Input: dimensioned drawing with shaded views. Units: mm. Origin: part minimum x, y, z. A direction names the side the tool comes from. Round coordinates to 2 decimals unless told otherwise and drop trailing zeros. Loops run counter-clockwise (first coordinate to the right, second up) from the corner with the lowest first, then second, coordinate; pieces in that order, holes last. Notation, with made-up numbers: (71.25, -3.75) - (115.25, -3.75) arc R16 cw to (115.25, 4.25) - close; hole circle Ø4 at (2, 44). An arc over 180 degrees is marked (long way). One line per question, with ' | ' between items.
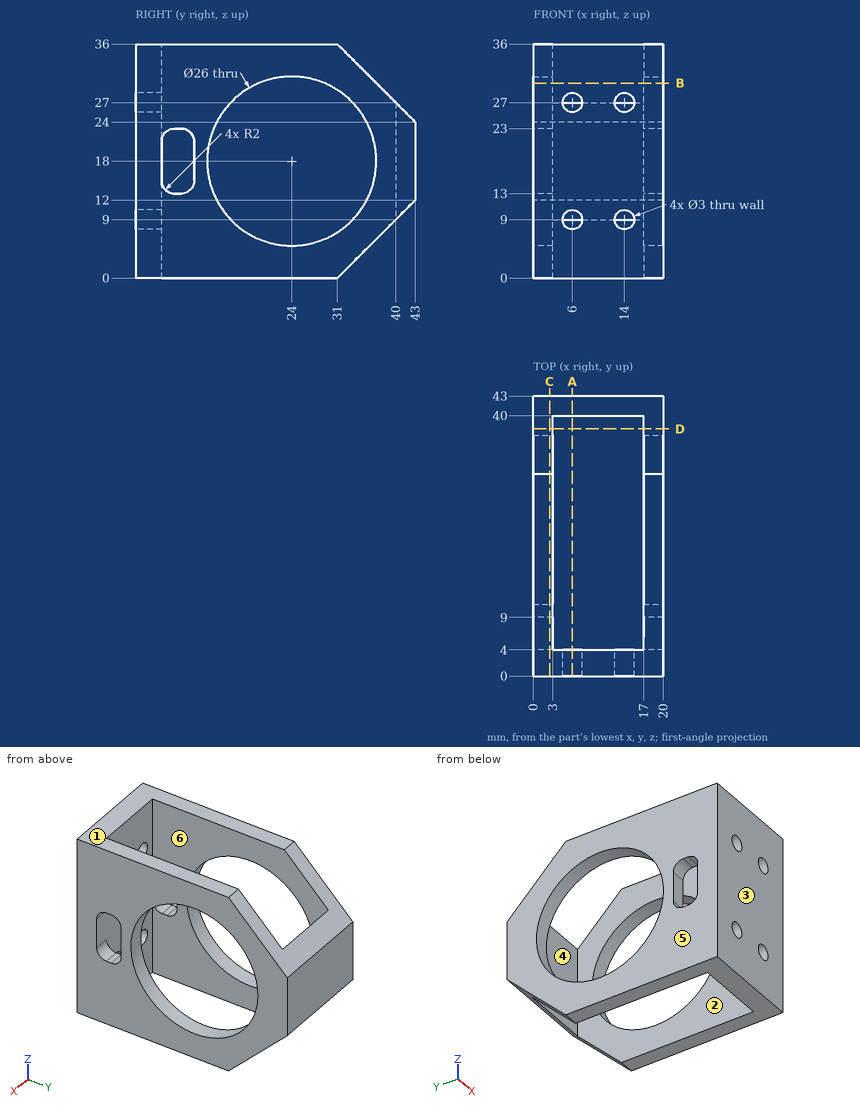
1. Section query B-B, the plane z = 30. Return loops of the section in (x, y), plus the area to 3 significant figures.
Worked out:
outline: (0, 0) - (20, 0) - (20, 19) - (17, 19) - (17, 4) - (3, 4) - (3, 19) - (0, 19) - close; (0, 29) - (3, 29) - (3, 37) - (0, 37) - close; (17, 29) - (20, 29) - (20, 37) - (17, 37) - close | area: 218 mm2
2. Section query D-D, the plane y = 38. Return loops of the section in (x, z), plus the area to 3 significant figures.
Worked out:
outline: (0, 7) - (3, 7) - (3, 29) - (0, 29) - close; (17, 7) - (20, 7) - (20, 29) - (17, 29) - close | area: 132 mm2
3. Material intervals for probe 1 along X at (y, z) = (1.4, 9); probe 2 along Y at (x, z) = (18.2, 18); probe 3 along Y at (x, z) = (11.5, 18), sorted ascending.
Worked out:
probe 1: x = 0 to 4.5, 7.5 to 12.5, 15.5 to 20 | probe 2: y = 0 to 4, 9 to 11, 37 to 43 | probe 3: y = 0 to 4, 40 to 43
4. Section query C-C, the plane x = 2.5. Return loops of the section in (y, z), plus the area to 3 significant figures.
Worked out:
outline: (0, 0) - (31, 0) - (43, 12) - (43, 24) - (31, 36) - (0, 36) - close; hole (4, 15) arc R2 ccw to (6, 13) - (7, 13) arc R2 ccw to (9, 15) - (9, 21) arc R2 ccw to (7, 23) - (6, 23) arc R2 ccw to (4, 21) - close; hole circle Ø26 at (24, 18) | area: 827 mm2
5. Mould query, pull axis Y, two halves, no side actions, for the marked faces 3, 4, 5 and 6. Classes: released by +Y, released by -Y, zero draft, split by the parting line, or undercut.
Worked out:
face 3: released by -Y | face 4: undercut | face 5: zero draft | face 6: undercut
6. Access query for the marked faces 1 and 2. Directions: +Z, -Z, +X, -X, +Y, -Y. A direction counts if a zero-diameter tool reaches every point of the face in a straight line with its end or side. Return the directions, or none.
Worked out:
face 1: +Z, +X, -X, +Y, -Y | face 2: +Z, -Z
7. Section query A-A, the plane x = 6. Return loops of the section in (y, z), plus the area to 3 significant figures.
Worked out:
outline: (0, 0) - (4, 0) - (4, 7.5) - (0, 7.5) - close; (0, 10.5) - (4, 10.5) - (4, 25.5) - (0, 25.5) - close; (0, 28.5) - (4, 28.5) - (4, 36) - (0, 36) - close; (40, 9) - (43, 12) - (43, 24) - (40, 27) - close | area: 165 mm2
8. Contact query for flat-ended pins moving along their axis: P1, Ø4, axis at x = 17, y = 34.5, coming from the -Z side; P2, Ø4, axis at x = 14, z = 9, coming from the +Y side; P3, Ø2.5, axis at x = 14, z = 27, coming from the -Y side. Output: stop coordinate, or through.
Worked out:
P1: stops at z = 1.5 | P2: stops at y = 42 | P3: stops at y = 40
